```python
from build123d import *

# Parameters (mm, degrees)
CROQUIS1_R              = 1.55
CROQUIS1_W              = 16
CROQUIS1_H              = 3.05
CROQUIS1_W_2            = 3.05
CROQUIS1_H_2            = 12
SALIENTE_EXTRUIR1_DEPTH = 3
CROQUIS2_R              = 1.4
CORTAR_EXTRUIR2_DEPTH   = 4


with BuildPart() as part:
    # Croquis1 → Saliente-Extruir1 (new body)
    with BuildSketch(Plane.XY):
        with BuildLine():
            Line((56, -21.3), (56, -44.5))
            ThreePointArc((56, -44.5), (55.707106781, -45.207106781), (55, -45.5))
            Line((55, -45.5), (-55, -45.5))
            ThreePointArc((-55, -45.5), (-55.707106781, -45.207106781), (-56, -44.5))
            Line((-56, -44.5), (-56, -21.15))
            ThreePointArc((-56, -21.15), (-55.707106781, -20.442893219), (-55, -20.15))
            Line((-55, -20.15), (-42, -20.15))
            ThreePointArc((-42, -20.15), (-41.292893219, -19.857106781), (-41, -19.15))
            Line((-41, -19.15), (-41, 35.1))
            ThreePointArc((-41, 35.1), (-41.292893219, 35.807106781), (-42, 36.1))
            Line((-42, 36.1), (-55, 36.1))
            ThreePointArc((-55, 36.1), (-55.707106781, 36.392893219), (-56, 37.1))
            Line((-56, 37.1), (-56, 44.5))
            ThreePointArc((-56, 44.5), (-55.707106781, 45.207106781), (-55, 45.5))
            Line((-55, 45.5), (55, 45.5))
            ThreePointArc((55, 45.5), (55.707106781, 45.207106781), (56, 44.5))
            Line((56, 44.5), (56, 37.1))
            ThreePointArc((56, 37.1), (55.707106781, 36.392893219), (55, 36.1))
            Line((55, 36.1), (41.2, 36.1))
            ThreePointArc((41.2, 36.1), (40.492893219, 35.807106781), (40.2, 35.1))
            Line((40.2, 35.1), (40.2, -19.3))
            ThreePointArc((40.2, -19.3), (40.492893219, -20.007106781), (41.2, -20.3))
            Line((41.2, -20.3), (55, -20.3))
            ThreePointArc((55, -20.3), (55.707106781, -20.592893219), (56, -21.3))
        make_face()
        with Locations((-35.5, 24.5)):
            Circle(CROQUIS1_R, mode=Mode.SUBTRACT)
        with Locations((-35.5, 14.5)):
            Circle(CROQUIS1_R, mode=Mode.SUBTRACT)
        with Locations((-35.5, -0.5)):
            Circle(CROQUIS1_R, mode=Mode.SUBTRACT)
        with Locations((-35.5, -10.5)):
            Circle(CROQUIS1_R, mode=Mode.SUBTRACT)
        with BuildLine():
            Line((-8.4, 39.9), (-22.5, 39.9))
            ThreePointArc((-22.5, 39.9), (-23.207106781, 39.607106781), (-23.5, 38.9))
            Line((-23.5, 38.9), (-23.5, -1.1))
            ThreePointArc((-23.5, -1.1), (-23.207106781, -1.807106781), (-22.5, -2.1))
            Line((-22.5, -2.1), (21, -2.1))
            ThreePointArc((21, -2.1), (21.707106781, -1.807106781), (22, -1.1))
            Line((22, -1.1), (22, 38.9))
            ThreePointArc((22, 38.9), (21.707106781, 39.607106781), (21, 39.9))
            Line((21, 39.9), (7.6, 39.9))
            Line((7.6, 39.9), (7.6, 42.95))
            Line((7.6, 42.95), (-8.4, 42.95))
            Line((-8.4, 42.95), (-8.4, 39.9))
        make_face(mode=Mode.SUBTRACT)
        with Locations((1.45, -41.525)):
            Rectangle(CROQUIS1_W, CROQUIS1_H, mode=Mode.SUBTRACT)
        with Locations((51.475, -28.3)):
            Rectangle(CROQUIS1_W_2, CROQUIS1_H_2, mode=Mode.SUBTRACT)
        with Locations((-51.475, -28.15)):
            Rectangle(CROQUIS1_W_2, CROQUIS1_H_2, mode=Mode.SUBTRACT)
    extrude(amount=SALIENTE_EXTRUIR1_DEPTH)

    # Croquis2 → Cortar-Extruir2 (cut, through all)
    with BuildSketch(Plane.XY.offset(3)):
        with Locations((53, 42)):
            Circle(CROQUIS2_R)
        with Locations((-52.5, 42)):
            Circle(CROQUIS2_R)
        with Locations((-52.5, -42)):
            Circle(CROQUIS2_R)
        with Locations((53, -42)):
            Circle(CROQUIS2_R)
    extrude(amount=-CORTAR_EXTRUIR2_DEPTH, mode=Mode.SUBTRACT)


solid = part.part
```
Design review of the part built by this model. Coordinates are the model's own, in mm. A direction names the side the tool comes from. Coordinates: 2 decimals unless noted, no trailing zeros. Order: outer loops, then holes, each group sorted by start corner. A loop starts at its lowest first (then second) coordinate and runs counter-clockwise, first axis right, second up. Notation, with made-up numbers: M 89.25,53.5 L 147.25,53.5 A6 ccw 147.25,57.5 Z; hole C -37,35.5 d7. An arc over 180 degrees is marked long. Answer as a JSON object with one key per item and string values. Group by question number.
1) Add section A-A, the plane x = 43. Write out the cut boundary in (y, z), then the cut area to 3 significant figures.
2) Wall thickness on L1, parallel to X at y = -23, z = 0.75; L2, parallel to Y at x = -52.5, z = 1.2; L3, parallel to Y at x = 44.5, z = 1.5: over which ranges is each line inside the solid? List them lowest first.
3) Mouldability with a two-part tool opening along X and no side actions: class faces 1 (the flat face through (-41, 8, 1)), 2 (the flat face through (14, 39.9, 1)), 3 (the flat face through (1, -9, 0)) as pulls with the +X half, pulls with the -X half, needs draft (parallel to the pull), parting line crosses it, or undercut.
4) Tool access review of faces 4 (the flat face through (51, -34.3, 1)), 5 (the flat face through (-1, 45.5, 1)), 6 (the flat face through (48, 36.1, 1)), 7 (the flat face through (56, -33, 1)), 8 (the flat face through (-48, 36.1, 1)): name each direction out of +Z, -Z, +X, -X, +Y, -Y from which nothing blocks a thin tool from reaching the whole face with its end or side.
5) Add section B-B, the plane y = -28.5. Write out the cut boundary in (x, z), then the cut area to 3 significant figures.
6) Add section C-C, the plane z = 0.6. Count the separate pieces of the cut face and the enclosed holes in it, then the cut area to 3 significant figures.
7) For pin 1 (1 mm diameter, centred on y = 33.5, z = 0.5, fed in from +X); pin 2 (1.5 mm diameter, centred on y = 15, z = 1, fed in from -X), all flat-tipped, find the tip position at first contact; note any pin that passes through.
Computed values:
{
 "1": {"outline": "M -45.5,0 L -20.3,0 L -20.3,3 L -45.5,3 Z; M 36.1,0 L 45.5,0 L 45.5,3 L 36.1,3 Z", "area": "104 mm^2"},
 "2": {"L1": "x = -56 to -53, -49.95 to 49.95, 53 to 56", "L2": "y = -45.5 to -43.4, -40.6 to -34.15, -22.15 to -20.15, 36.1 to 40.6, 43.4 to 45.5", "L3": "y = -45.5 to -20.3, 36.1 to 45.5"},
 "3": {"face 1": "pulls with the -X half", "face 2": "undercut", "face 3": "needs draft"},
 "4": {"face 4": "+Z, -Z", "face 5": "+Z, -Z, +X, -X, +Y", "face 6": "+Z, -Z, +X", "face 7": "+Z, -Z, +X, +Y, -Y", "face 8": "+Z, -Z, -X"},
 "5": {"outline": "M -56,0 L -53,0 L -53,3 L -56,3 Z; M -49.95,0 L 49.95,0 L 49.95,3 L -49.95,3 Z; M 53,0 L 56,0 L 56,3 L 53,3 Z", "area": "318 mm^2"},
 "6": {"separate pieces": "1", "enclosed holes": "12", "area": "6,320 mm^2"},
 "7": {"pin 1": "stops at x = 40.2", "pin 2": "stops at x = -41"}
}
